The model under review builds one solid part; all positions refer to its coordinate system, in mm. A direction names the side the tool comes from. Coordinates: 2 decimals unless noted, no trailing zeros. Write each loop counter-clockwise with the first axis right and the second up, starting at its lowest first coordinate (ties: lowest second). Pieces come first, ordered by that corner, then holes. Notation, with made-up numbers: (18, -37) - (74, -37) arc R20 cw to (74, -16) - close; hole circle Ø8 at (78, -0.75). An arc over 180 degrees is marked (long way). Put each result on its own line as item: value. Start each with the question number.
Item 1: To check wall thickness, follow L1, parallel to Y at x = 0, z = 16.5; L2, parallel to X at y = 0, z = 13; L3, parallel to Y at x = 4, z = 4.5. State the ranges of each line that lie inside material, in increasing order. Write a range as [from, to].
Item 2: Mouldability with a two-part tool opening along Z and no side actions: class faces 1 (the face through (2, 2, 25)), 2 (the face through (-1, -5, 0)), 3 (the face through (-3.233, 1.341, 16.845)) as pulls with the +Z half, pulls with the -Z half, needs draft (parallel to the pull), parting line crosses it, or undercut.
Item 3: For pin 1 (4.5 mm diameter, centred on x = 0, y = 0, fed in from +Z); pin 2 (5 mm diameter, centred on y = -3.5, z = 21, fed in from -X); pin 3 (1.5 mm diameter, centred on x = -4, y = -4.5, fed in from +Z); pin 4 (4 mm diameter, centred on y = -5, z = 16, fed in from +X), all flat-tipped, find the tip position at first contact; note any pin that passes through.
Item 4: Machinability: for faces 4 (the face through (2.706, -2.482, 15.687)), 5 (the face through (-5.96, -1.88, 6.46)), which of the approach directions +Z, -Z, +X, -X, +Y, -Y give a long, thin tool a straight path to every point of the face, cutting with its end or side? Answer none if there is none.
Item 5: Consider section B-B on x = 4.75. State how many separate pieces and enclosed holes the cut face has, then the cut area to 3 significant figures.
Item 6: Consider section A-A on z = 9. Give the boundary of the cut face in (x, y).
```python
from build123d import *

# Parameters (mm, degrees)
F4_R     = 2.5
F5_DEPTH = 25.001


with BuildPart() as f1:
    # F0 (on Front) → F1 (revolve)
    with BuildSketch(Plane.XZ):
        with BuildLine():
            Line((-6.25, 13.108572), (-6.25, 0))
            Line((-6.25, 0), (0, 0))
            Line((0, 0), (0, 25))
            Line((0, 25), (-3.5, 25))
            ThreePointArc((-3.5, 25), (-5, 21.429286), (-3.5, 17.858572))
            Line((-3.5, 17.858572), (-3.5, 15.858572))
            Line((-3.5, 15.858572), (-6.25, 13.108572))
        make_face()
    revolve(axis=Axis((0, 0, 12.5), (0, 0, 1)))

    # F2 (on Front) → F3 (revolve, cut)
    with BuildSketch(Plane.XZ):
        with BuildLine():
            Line((0, 0), (0, 7.291288))
            ThreePointArc((0, 7.291288), (-3.535534, 5.826822), (-5, 2.291288))
            ThreePointArc((-5, 2.291288), (-4.859037, 1.112408), (-4.444097, 0))
            Line((-4.444097, 0), (0, 0))
        make_face()
        with BuildLine():
            ThreePointArc((-5, 2.291288), (-3.535534, 5.826822), (0, 7.291288))
            Line((0, 7.291288), (0, 10.291288))
            ThreePointArc((0, 10.291288), (-3.647185, 7.008278), (-5, 2.291288))
        make_face()
        with BuildLine():
            ThreePointArc((-4.444097, 0), (-4.859037, 1.112408), (-5, 2.291288))
            ThreePointArc((-5, 2.291288), (-4.924681, 1.135866), (-4.7, 0))
            Line((-4.7, 0), (-4.444097, 0))
        make_face()
    revolve(axis=Axis((0, 0, 2.291288), (0, 0, 1)), mode=Mode.SUBTRACT)

    # F4 (on face) → F5 (cut, through all)
    with BuildSketch(Plane.XY.offset(25)):
        Circle(F4_R)
    extrude(amount=-F5_DEPTH, mode=Mode.SUBTRACT)


solid = f1.part
```
Report:
1. L1: [-3.5, -2.5], [2.5, 3.5]
1. L2: [-6.25, -2.5], [2.5, 6.25]
1. L3: [-4.8, -2.51], [2.51, 4.8]
2. face 1: pulls with the +Z half
2. face 2: pulls with the -Z half
2. face 3: undercut
3. pin 1: through
3. pin 2: x = -4.89
3. pin 3: z = 14.09
3. pin 4: x = 3.19
4. face 4: none
4. face 5: +Z, -Z
5. separate pieces: 2
5. enclosed holes: 1
5. area: 112 mm²
6. outline: circle Ø12.5 at (0, 0); hole circle Ø5 at (0, 0)
